The model under review builds one solid part; all positions refer to its coordinate system, in mm. Coordinates: 2 decimals unless noted, no trailing zeros. Loops run counter-clockwise (first coordinate to the right, second up) from the corner with the lowest first, then second, coordinate; pieces in that order, holes last. Notation, with made-up numbers: (-20, 50) - (24, 50) arc R24 ccw to (24, 65) - close; hole circle Ø9 at (53.25, 15.5). An arc over 180 degrees is marked (long way). Answer in a Markdown table with one row per item. Add a question column.
(1) For line 1 along Y through (x, z) = (25.4, 4.5) (3 decimals); line 2 along X through (y, z) = (50, 1), list the stretches that pass through material, from the lowest coordinate up.
(2) We need section A-A on y = 44.45. Write out the cut boundary in (x, z) (3 decimals), plus the area to 3 significant figures.
(3) Mouldability with a two-part tool opening along X and no side actions: class faces 1 (the flat face through (-2, 1, 9.525)), 2 (the flat face through (152.4, -1, 5)), 3 (the cylindrical face through (18.231, 55.694, 4.696)) as +X half, -X half, draft (parallel to the pull), parting line (faces both ways), or undercut.
(4) We need section B-B on x = 25.4. Write out the cut boundary in (y, z) (3 decimals).
from build123d import *

# Parameters (mm, degrees)
SKETCH1_W                     = 304.8
SKETCH1_H                     = 152.4
BOSS_EXTRUDE1_DEPTH           = 9.525
SKETCH5_R                     = 13.335
CUT_EXTRUDE3_DEPTH            = 171.65440406
F_1_1_05_DIAMETER_HOLE1_D     = 26.67
F_1_1_05_DIAMETER_HOLE1_DEPTH = 60.324
F_1_1_05_DIAMETER_HOLE1_TIP   = 8.012476355
F_1_1_05_DIAMETER_HOLE2_D     = 26.67
F_1_1_05_DIAMETER_HOLE2_DEPTH = 60.324
F_1_1_05_DIAMETER_HOLE2_TIP   = 8.012476355


with BuildPart() as part:
    # Sketch1 → Boss-Extrude1 (new body)
    with BuildSketch(Plane.XY):
        Rectangle(SKETCH1_W, SKETCH1_H)
    extrude(amount=BOSS_EXTRUDE1_DEPTH)

    # Sketch5 → Cut-Extrude3 (cut, through all)
    with BuildSketch(Plane(origin=(0, 0, 0), x_dir=(-1, 0, 0), z_dir=(0, 0, -1))):
        with Locations((-25.4, 44.45)):
            Circle(SKETCH5_R)
    extrude(amount=-CUT_EXTRUDE3_DEPTH, mode=Mode.SUBTRACT)

    # 1 (1.05) Diameter Hole1
    with Locations(Plane(origin=(1137.132872188, -76.2, 69.85), x_dir=(1, 0, 0), z_dir=(0, 0, 1))):
        with Locations((-1111.732872188, 120.65)):
            Hole(F_1_1_05_DIAMETER_HOLE1_D / 2, depth=F_1_1_05_DIAMETER_HOLE1_DEPTH)
            with Locations((0, 0, -(F_1_1_05_DIAMETER_HOLE1_DEPTH + F_1_1_05_DIAMETER_HOLE1_TIP / 2))):  # 118° drill point
                Cone(0, F_1_1_05_DIAMETER_HOLE1_D / 2, F_1_1_05_DIAMETER_HOLE1_TIP, mode=Mode.SUBTRACT)

    # 1 (1.05) Diameter Hole2
    with Locations(Plane(origin=(1137.132872188, -76.2, 9.525), x_dir=(1, 0, 0), z_dir=(0, 0, 1))):
        with Locations((-1111.732872188, 120.65)):
            Hole(F_1_1_05_DIAMETER_HOLE2_D / 2, depth=F_1_1_05_DIAMETER_HOLE2_DEPTH)
            with Locations((0, 0, -(F_1_1_05_DIAMETER_HOLE2_DEPTH + F_1_1_05_DIAMETER_HOLE2_TIP / 2))):  # 118° drill point
                Cone(0, F_1_1_05_DIAMETER_HOLE2_D / 2, F_1_1_05_DIAMETER_HOLE2_TIP, mode=Mode.SUBTRACT)


solid = part.part
Outcome:
| question | item | result |
|---|---|---|
| 1 | line 1 | -76.2 to 31.115, 57.785 to 76.2 |
| 1 | line 2 | -152.4 to 13.27, 37.53 to 152.4 |
| 2 | outline | (-152.4, 0) - (12.065, 0) - (12.065, 9.525) - (-152.4, 9.525) - close; (38.735, 0) - (152.4, 0) - (152.4, 9.525) - (38.735, 9.525) - close |
| 2 | area | 2,650 mm² |
| 3 | face 1 | draft |
| 3 | face 2 | +X half |
| 3 | face 3 | undercut |
| 4 | outline | (-76.2, 0) - (31.115, 0) - (31.115, 9.525) - (-76.2, 9.525) - close; (57.785, 0) - (76.2, 0) - (76.2, 9.525) - (57.785, 9.525) - close |
